from build123d import *

# Parameters (mm, degrees)
BOSS_EXTRUDE1_DEPTH   = 10
SKETCH1_R             = 22.5
BOSS_EXTRUDE1_2_DEPTH = 10
BOSS_EXTRUDE6_DEPTH   = 10
SKETCH4_R             = 2.5
CUT_EXTRUDE1_DEPTH    = 234.806009457


with BuildPart() as part:
    # Sketch1 → Boss-Extrude1 (new body)
    with BuildSketch(Plane(origin=(0, 0, 0), x_dir=(1, 0, 0), z_dir=(0, 1, 0))):
        with BuildLine():
            Line((-25.5, 6), (-25.5, 0))
            ThreePointArc((-25.5, 0), (-25.315717118, -3.06014163), (-24.765532016, -6.076053321))
            Line((-24.765532016, -6.076053321), (-20, -25.5))
            add(Edge.make_bspline(
                [(-20, -25.5), (-10.418058305, -61.939732527), (-10, -99)],
                knots=[0, 0, 0, 0.916388339, 0.916388339, 0.916388339], degree=2))
            Line((-10, -99), (0, -99))
            Line((0, -99), (0, -172.5))
            Line((0, -172.5), (10, -172.5))
            Line((10, -172.5), (10, -105.767954903))
            add(Edge.make_bspline(
                [(10, -99), (9.961856183, -102.381394532), (10, -105.767954903)],
                knots=[0.916388339, 0.916388339, 0.916388339, 1, 1, 1], degree=2))
            add(Edge.make_bspline(
                [(20, -25.5), (10.418058305, -61.939732527), (10, -99)],
                knots=[0, 0, 0, 0.916388339, 0.916388339, 0.916388339], degree=2))
            Line((20, -25.5), (24.765532016, -6.076053321))
            ThreePointArc((24.765532016, -6.076053321), (25.315717118, -3.06014163), (25.5, 0))
            Line((25.5, 0), (25.5, 6))
            Line((25.5, 6), (15.5, 6))
            Line((15.5, 6), (15.5, 0))
            ThreePointArc((15.5, 0), (0, -15.5), (-15.5, 0))
            Line((-15.5, 0), (-15.5, 6))
            Line((-15.5, 6), (-25.5, 6))
        make_face()
    extrude(amount=BOSS_EXTRUDE1_DEPTH)



with BuildPart() as body_2:
    # Sketch1 → Boss-Extrude1 2 (new body)
    with BuildSketch(Plane(origin=(0, 0, 0), x_dir=(1, 0, 0), z_dir=(0, 1, 0))):
        with BuildLine():
            Line((-10, -172.5), (-10, -99))
            add(Edge.make_bspline(
                [(-20, -172.5), (-10.418058305, -136.060267473), (-10, -99)],
                knots=[0, 0, 0, 0.916388339, 0.916388339, 0.916388339], degree=2))
            Line((-20, -172.5), (-25.5, -189.704369859))
            ThreePointArc((-25.5, -189.704369859), (15.380509925, -222.796708412), (0, -172.5))
            Line((0, -172.5), (-10, -172.5))
        make_face()
        with Locations(Location((0, -200, 0), (0, 0, 270))):
            Circle(SKETCH1_R, mode=Mode.SUBTRACT)
    extrude(amount=BOSS_EXTRUDE1_2_DEPTH)


with BuildPart() as part_1:
    add(part.part)

    add(body_2.part)  # Boss-Extrude6 merges body 2
    # Sketch3 → Boss-Extrude6 (add)
    with BuildSketch(Plane(origin=(0, 10, 0), x_dir=(1, 0, 0), z_dir=(0, 1, 0))):
        with BuildLine():
            ThreePointArc((0, -172.5), (5.087835239, -172.974753792), (10, -174.382623085))
            Line((10, -174.382623085), (10, -99))
            Line((10, -99), (-10, -99))
            Line((-10, -99), (-10, -172.5))
            Line((-10, -172.5), (0, -172.5))
        make_face()
        with BuildLine():
            Line((10, -99), (10, -174.382623085))
            ThreePointArc((10, -174.382623085), (19.332653234, -180.442430648), (25.5, -189.704369859))
            add(Edge.make_bspline(
                [(25.5, -189.704369859), (10.530956194, -144.964559023), (10, -99)],
                knots=[0, 0, 0, 0.931489523, 0.931489523, 0.931489523], degree=2))
        make_face()
    extrude(amount=-BOSS_EXTRUDE6_DEPTH)

    # Sketch4 → Cut-Extrude1 (cut, through all)
    with BuildSketch(Plane.ZY.offset(25.5)):
        with Locations((-3, 7)):
            Circle(SKETCH4_R)
    extrude(amount=-CUT_EXTRUDE1_DEPTH, mode=Mode.SUBTRACT)


solid = part_1.part
For this review, take the finished solid that the model builds, in its own axes (mm). A direction names the side the tool comes from. Round coordinates to 2 decimals unless told otherwise and drop trailing zeros. Write each loop counter-clockwise with the first axis right and the second up, starting at its lowest first coordinate (ties: lowest second). Pieces come first, ordered by that corner, then holes. Notation, with made-up numbers: (17, 81) - (60, 81) arc R16 cw to (60, 105) - close; hole circle Ø3 at (53.5, 70.5). An arc over 180 degrees is marked (long way). Write item = value, one per line. Start each with the question number.
1. Consider section B-B on z = 200. State the section outline as (x, y) points.
2. Draft analysis for pull direction Z (two halves, no side actions). For faces 1 (the face through (0, 10, 83)), 2 (the face through (20.43, 4.78, -1.85)), 3 (the face through (-0.75, 4.93, 227.49)), state which applies: released by +Z, released by -Z, zero draft, split by the parting line, or undercut.
3. Consider section C-C on x = -2. State the section outline as (y, z) points.
4. Wall thickness on L1, parallel to Y at x = 20, z = -3; L2, parallel to X at y = 4.5, z = 214.5; L3, parallel to X at y = 5.25, z = 215.5: over which ranges is each line inside the solid? List them lowest first.
5. Consider section A-A on z = -3. State the section outline as (x, y) points.
6. For pin 1 Ø3 at (y, z) = (4, -3.5) entering from +X; pin 2 Ø1.5 at (x, y) = (-17.5, 3) entering from +Z; pin 3 Ø1.5 at (x, y) = (3, 3) entering from -Z; pin 4 Ø5 at (x, z) = (18, 188.5) entering from -Y, all flat-tipped, find the tip position at first contact; note any pin that passes through.
7. For faces 4 (the face through (25.5, 4, -3)), 5 (the face through (-25.5, 4, -3)), 6 (the face through (15.5, 4, -3)), 7 (the face through (-22.416, 4.93, 15.652)), list the 3-axis set-ups (+Z, -Z, +X, -X, +Y, -Y) from which the entire face can be reached by the end or side of a thin tool; tool diameter is ignored.
Evaluation:
q1.outline = (-27.5, 0) - (-22.5, 0) - (-22.5, 10) - (-27.5, 10) - close; (22.5, 0) - (27.5, 0) - (27.5, 10) - (22.5, 10) - close
q2.face_1 = zero draft
q2.face_2 = undercut
q2.face_3 = split by the parting line
q3.outline = (0, 15.37) - (10, 15.37) - (10, 177.59) - (0, 177.59) - close; (0, 222.41) - (10, 222.41) - (10, 227.43) - (0, 227.43) - close
q4.L1 = 0 to 4.5, 9.5 to 10
q4.L2 = -23.37 to -17.2, 17.2 to 23.37
q4.L3 = -22.72 to -16.31, 16.31 to 22.72
q5.outline = (-25.5, 0) - (-15.5, 0) - (-15.5, 4.5) - (-25.5, 4.5) - close; (-25.5, 9.5) - (-15.5, 9.5) - (-15.5, 10) - (-25.5, 10) - close; (15.5, 0) - (25.5, 0) - (25.5, 4.5) - (15.5, 4.5) - close; (15.5, 9.5) - (25.5, 9.5) - (25.5, 10) - (15.5, 10) - close
q6.pin_1 = 25.5
q6.pin_2 = 221.81
q6.pin_3 = 15.04
q6.pin_4 = 0
q7.face_4 = -Z, +X, +Y, -Y
q7.face_5 = -Z, -X, +Y, -Y
q7.face_6 = -Z, +Y, -Y
q7.face_7 = -X, +Y, -Y
